from build123d import *

# Parameters (mm, degrees)
SKETCH1_W           = 20
SKETCH1_H           = 20
BOSS_EXTRUDE1_DEPTH = 20
SKETCH2_R           = 6
CUT_EXTRUDE1_DEPTH  = 21
CUT_EXTRUDE2_DEPTH  = 21
SKETCH4_W           = 30
SKETCH4_H           = 80
BOSS_EXTRUDE2_DEPTH = 27


with BuildPart() as part:
    # Sketch1 → Boss-Extrude1 (new body)
    with BuildSketch(Plane.XY):
        Rectangle(SKETCH1_W, SKETCH1_H)
    extrude(amount=BOSS_EXTRUDE1_DEPTH)

    # Sketch2 → Cut-Extrude1 (cut, through all)
    with BuildSketch(Plane(origin=(0, 10, 0), x_dir=(1, 0, 0), z_dir=(0, 1, 0))):
        with Locations((0, -10)):
            Circle(SKETCH2_R)
    extrude(amount=-CUT_EXTRUDE1_DEPTH, mode=Mode.SUBTRACT)

    # Sketch3 → Cut-Extrude2 (cut, through all)
    with BuildSketch(Plane(origin=(0, 10, 0), x_dir=(1, 0, 0), z_dir=(0, 1, 0))):
        with BuildLine():
            Line((-10, -12.714318114), (-10, -20))
            Line((-10, -20), (-3.788282588, -20))
            add(Edge.make_bspline(
                [(-10, -12.714318114), (-5.112714727, -14.756625636), (-3.788282588, -20)],
                knots=[0, 0, 0, 1, 1, 1], degree=2))
        make_face()
        with BuildLine():
            Line((10, -12.714318114), (10, -20))
            Line((10, -20), (3.788282588, -20))
            add(Edge.make_bspline(
                [(10, -12.714318114), (5.112714727, -14.756625636), (3.788282588, -20)],
                knots=[0, 0, 0, 1, 1, 1], degree=2))
        make_face()
    extrude(amount=-CUT_EXTRUDE2_DEPTH, mode=Mode.SUBTRACT)

    # Sketch4 → Boss-Extrude2 (add)
    with BuildSketch(Plane(origin=(0, 0, 0), x_dir=(-1, 0, 0), z_dir=(0, 0, -1))):
        Rectangle(SKETCH4_W, SKETCH4_H)
    extrude(amount=BOSS_EXTRUDE2_DEPTH)


solid = part.part
Part model, mm, in its own coordinate system. A direction names the side the tool comes from. Round coordinates to 2 decimals unless told otherwise and drop trailing zeros. Order: outer loops, then holes, each group sorted by start corner. A loop starts at its lowest first (then second) coordinate and runs counter-clockwise, first axis right, second up. Notation, with made-up numbers: (67, 5.25) -> (83, 5.25) arc R33 ccw to (83, 40.25) -> close; hole circle Ø7 at (-15, 58.5). An arc over 180 degrees is marked (long way). Put each result on its own line as item: value.
Q1. Tool access for faces 4 (the face through (0, 10, 3)), 5 (the face through (0, -10, 3)), 6 (the face through (-10, 0, 6)), 7 (the face through (0, 1, -27)), 8 (the face through (0, 0, 20)): list every direction of +Z, -Z, +X, -X, +Y, -Y with a clear straight run to the whole face (end or side of a thin tool).
From the geometry:
face 4: +Z, +X, -X, +Y
face 5: +Z, +X, -X, -Y
face 6: +Z, -X, +Y, -Y
face 7: -Z, +X, -X, +Y, -Y
face 8: +Z, +X, -X, +Y, -Y
Q2. Pull direction X, two halves, no side cores. Call faces 1 (the face through (-0.78, 0.14, 4.05)), 2 (the face through (0, 40, -13)), 3 (the face through (10, 0, 6)): pulls with the +X half, pulls with the -X half, needs draft (parallel to the pull), parting line crosses it, or undercut.
From the geometry:
face 1: undercut
face 2: needs draft
face 3: pulls with the +X half
Q3. Wall check: line 1 (X direction, y = -1.25, z = 10); line 2 (Z direction, x = 0, y = -5); line 3 (Z direction, x = -10.5, y = -34). Give the ranges that are in metal, low to high. Write a range as [from, to].
From the geometry:
line 1: x = [-10, -6], [6, 10]
line 2: z = [-27, 4], [16, 20]
line 3: z = [-27, 0]
Q4. Band-saw the part on C-C (y = 31). Give the cut face in (x, z), and give its area (3 significant figures).
From the geometry:
outline: (-15, -27) -> (15, -27) -> (15, 0) -> (-15, 0) -> close
area: 810 mm2
Q5. Band-saw the part on B-B (x = 0). Give the cut face in (y, z).
From the geometry:
outline: (-40, -27) -> (40, -27) -> (40, 0) -> (10, 0) -> (10, 4) -> (-10, 4) -> (-10, 0) -> (-40, 0) -> close; (-10, 16) -> (10, 16) -> (10, 20) -> (-10, 20) -> close
Q6. Pin check, flat tips, straight feed: pin 1 Ø14 at (y, z) = (-0.5, 5) entering from +X; pin 2 Ø10 at (x, y) = (6.5, -30) entering from +Z; pin 3 Ø11 at (x, z) = (0, 10) entering from +Y; pin 4 Ø6.5 at (y, z) = (2.5, 4) entering from -X. Stop position of each tip, or through.
From the geometry:
pin 1: stops at x = 15
pin 2: stops at z = 0
pin 3: passes through
pin 4: stops at x = -10
Q7. Band-saw the part on A-A (z = 10). Give the cut face in (x, y), and give its area (3 significant figures).
From the geometry:
outline: (-10, -10) -> (-6, -10) -> (-6, 10) -> (-10, 10) -> close; (6, -10) -> (10, -10) -> (10, 10) -> (6, 10) -> close
area: 160 mm2
Q8. Band-saw the part on D-D (x = -12). Give the cut face in (y, z).
From the geometry:
outline: (-40, -27) -> (40, -27) -> (40, 0) -> (-40, 0) -> close
